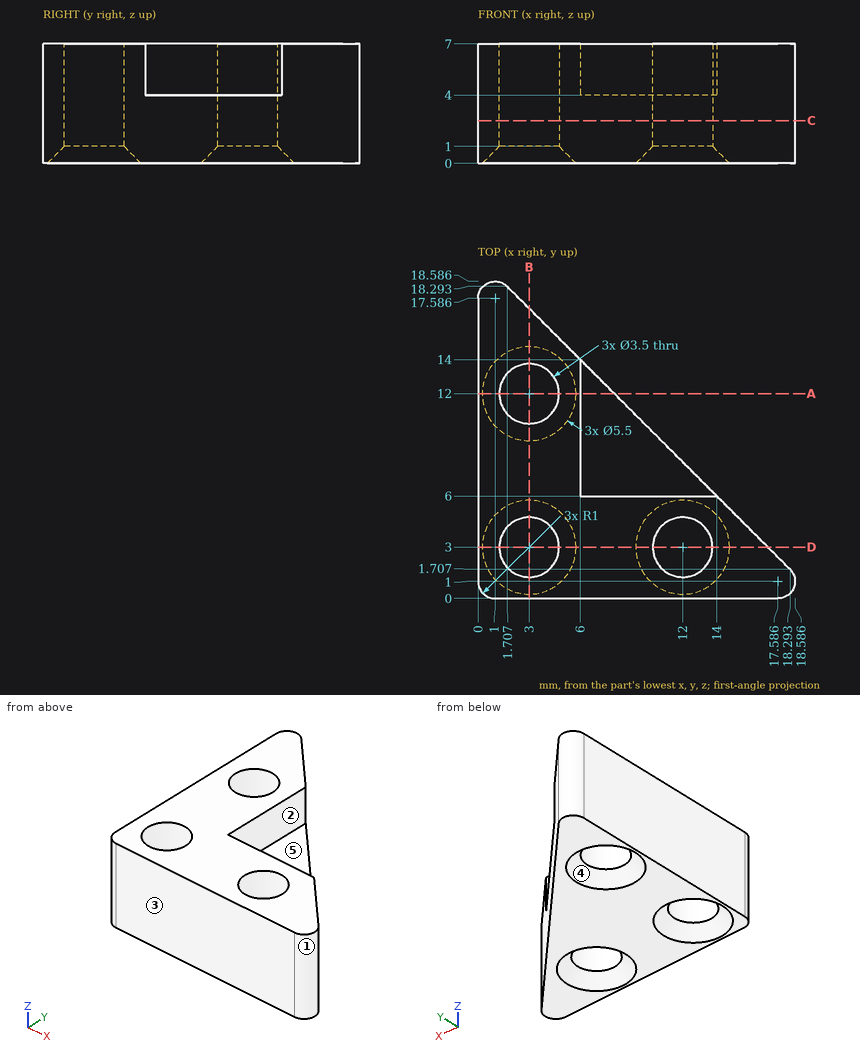
Here's the drawing with two shaded views (mm, measured from the low corner). I have some questions. A direction names the side the tool comes from. Round coordinates to 2 decimals unless told otherwise and drop trailing zeros. Write each loop counter-clockwise with the first axis right and the second up, starting at its lowest first coordinate (ties: lowest second). Pieces come first, ordered by that corner, then holes. Notation, with made-up numbers: M -17.75,89 L -9.75,89 A27 cw -9.75,122 Z; hole C -15,70 d11. An arc over 180 degrees is marked long. Answer in a Markdown table with one row per item. Add a question column.
Q1. Will these pins go through, and if not, where does the flat tip stop? pin 1 Ø2 at (y, z) = (2.5, 5) entering from +X; pin 2 Ø2.5 at (x, y) = (9, 11.5) entering from +Z; pin 3 Ø4 at (x, z) = (15, 6) entering from +Y.
Q2. On a 3-axis mill with a long thin cutter (end or side, diameter ignored), from which of +Z, -Z, +X, -X, +Y, -Y can I reach the whole of each face in a straight line? I mean the marked faces 1 and 2. Say none if no direction works.
Q3. Imagine slicing it at A-A (y = 12). Please give me the cut outline in (x, z).
Q4. Imagine slicing it at B-B (x = 3). Please give me the cut outline in (y, z).
Q5. If we mould it in two halves opening along Y, with no side actions, what happens to the marked faces 3, 4 and 5? For each: +Y half, -Y half, draft (parallel to the pull), parting line (faces both ways), or undercut.
Q6. Imagine slicing it at C-C (z = 2.5). Please give me the cut outline in (x, y), then the cut area to 3 significant figures.
Q7. If I drill on line 1 (Y direction, x = 4.5, z = 4.5); line 2 (Y direction, x = 3, z = 4.8); line 3 (X direction, y = 3.25, z = 2.5), over which ranges is the centre line in solid material (lowest first)? Write a range as from..to.
Values:
| question | item | result |
|---|---|---|
| 1 | pin 1 | x = 18.45 |
| 1 | pin 2 | z = 4 |
| 1 | pin 3 | y = 6 |
| 2 | face 1 | +Z, -Z, +X |
| 2 | face 2 | +Z, +X, +Y |
| 3 | outline | M 0,0 L 0.25,0 L 1.25,1 L 1.25,7 L 0,7 Z; M 4.75,1 L 5.75,0 L 8,0 L 8,4 L 6,4 L 6,7 L 4.75,7 Z |
| 4 | outline | M 0,0 L 0.25,0 L 1.25,1 L 1.25,7 L 0,7 Z; M 4.75,1 L 5.75,0 L 9.25,0 L 10.25,1 L 10.25,7 L 4.75,7 Z; M 13.75,1 L 14.75,0 L 17,0 L 17,7 L 13.75,7 Z |
| 5 | face 3 | -Y half |
| 5 | face 4 | undercut |
| 5 | face 5 | draft |
| 6 | outline | M 0,1 A1 ccw 1,0 L 17.59,0 A1 ccw 18.29,1.71 L 1.71,18.29 A1 ccw 0,17.59 Z; hole C 3,3 d3.5; hole C 3,12 d3.5; hole C 12,3 d3.5 |
| 6 | area | 168 mm^2 |
| 7 | line 1 | 0..2.1, 3.9..11.1, 12.9..15.5 |
| 7 | line 2 | 0..1.25, 4.75..10.25, 13.75..17 |
| 7 | line 3 | 0..1.27, 4.73..10.27, 13.73..16.75 |
